Check sheet for the drawn part. Datum: minimum x, y, z corner. Units: mm. Give positions to 0.01 mm unless a question says otherwise; leave off trailing zeros. Write each loop counter-clockwise with the first axis right and the second up, starting at its lowest first coordinate (ties: lowest second). Pieces come first, ordered by that corner, then holes. Notation, with made-up numbers: (22, 36.5) - (32, 36.5) arc R28 ccw to (32, 65.5) - close; hole circle Ø5 at (1.5, 39). An arc over 180 degrees is marked (long way). Use a Markdown table: item, result.
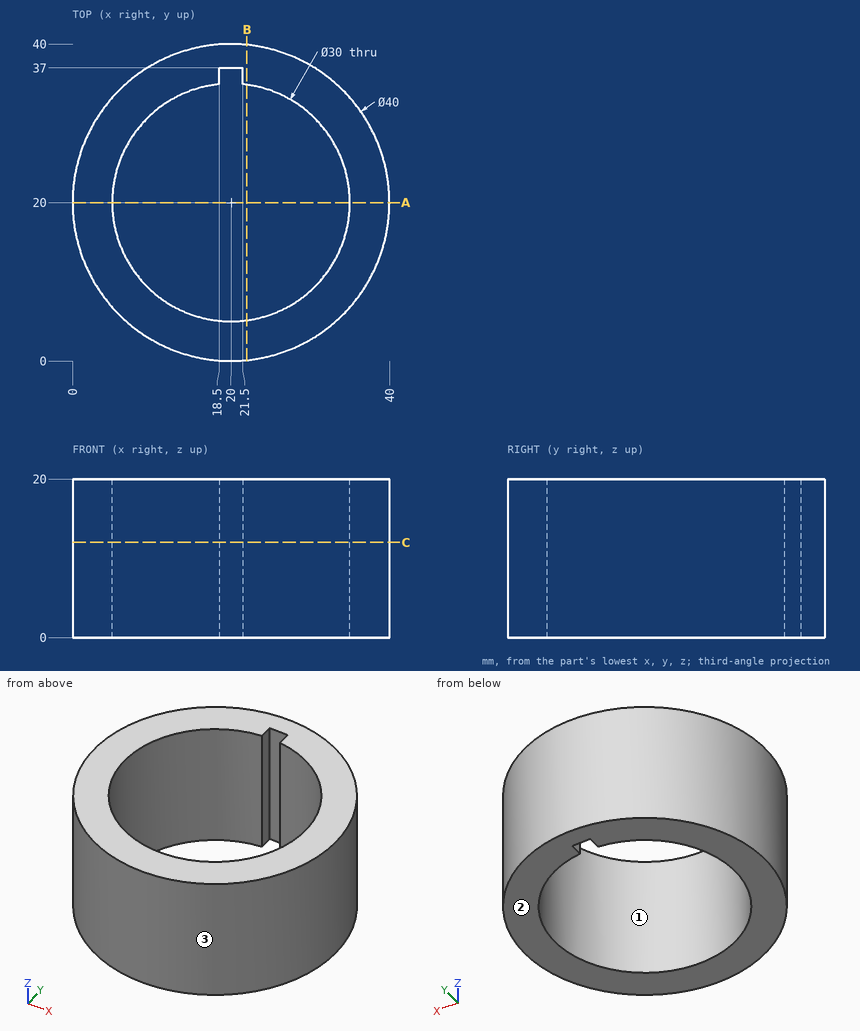
1) Mould release check, pull along Y, two halves, no side actions. Record for the marked faces 1, 2 and 3: pulls with the +Y half, pulls with the -Y half, needs draft (parallel to the pull), parting line crosses it, or undercut.
Working result:
| item | result |
|---|---|
| face 1 | undercut |
| face 2 | needs draft |
| face 3 | parting line crosses it |
2) Material ranges on L1, parallel to Y at x = 20, z = 4.5; L2, parallel to X at y = 27.5, z = 17.75; L3, parallel to Y at x = 10, z = 7.25, recorded low to high. Write a range as from..to.
Working result:
| item | result |
|---|---|
| L1 | y = 0..5, 37..40 |
| L2 | x = 1.46..7.01, 32.99..38.54 |
| L3 | y = 2.68..8.82, 31.18..37.32 |
3) Depth check by flat-ended pin: P1, Ø0.6, axis at y = 35.5, z = 6.5, coming from the +X side; P2, Ø0.9, axis at x = 19.5, z = 8.5, coming from the -Y side; P3, Ø3, axis at y = 17, z = 5, coming from the -X side; P4, Ø18, axis at x = 20, y = 20, coming from the -Z side. Enter the tip coordinate at first touch or a pass-through.
Working result:
| item | result |
|---|---|
| P1 | stops at x = 33 |
| P2 | stops at y = 0 |
| P3 | stops at x = 0.06 |
| P4 | passes through |
4) Section check B-B on x = 22. Record the boundary of the cut face in (y, z), then the cut area to 3 significant figures.
Working result:
| item | result |
|---|---|
| outline | (0.1, 0) - (5.13, 0) - (5.13, 20) - (0.1, 20) - close; (34.87, 0) - (39.9, 0) - (39.9, 20) - (34.87, 20) - close |
| area | 201 mm² |
5) Section check A-A on y = 20. Record the boundary of the cut face in (x, z).
Working result:
| item | result |
|---|---|
| outline | (0, 0) - (5, 0) - (5, 20) - (0, 20) - close; (35, 0) - (40, 0) - (40, 20) - (35, 20) - close |
6) Section check C-C on z = 12. Record the boundary of the cut face in (x, y).
Working result:
| item | result |
|---|---|
| outline | circle Ø40 at (20, 20); hole (18.5, 34.92) arc R15 ccw (long way) to (21.5, 34.92) - (21.5, 37) - (18.5, 37) - close |
